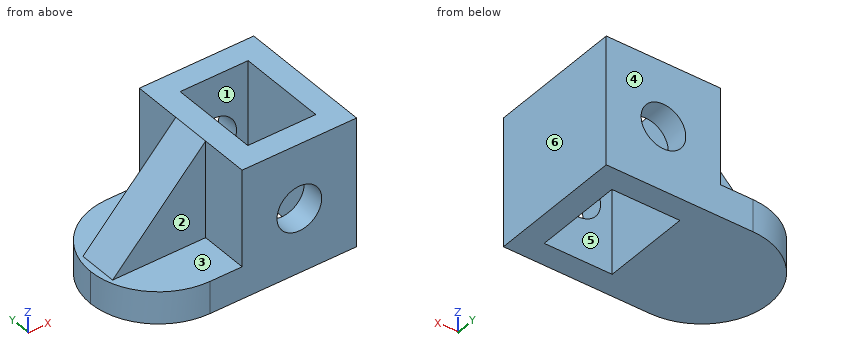
```python
from build123d import *

# Parameters (mm, degrees)
F0_R     = 12.5
F1_DEPTH = 76
F2_W     = 38
F2_H     = 50
F3_DEPTH = 124
F5_DEPTH = 125.4
F7_DEPTH = 54
F9_DEPTH = 25


with BuildPart() as f1:
    # F0 (on Front) → F1 (new body)
    with BuildSketch(Plane.XZ):
        Polygon((0, 18), (0, 0), (120, 0), (120, 72), (56, 72), (56, 18), align=None)
        with Locations((88, 36)):
            Circle(F0_R, mode=Mode.SUBTRACT)
    extrude(amount=F1_DEPTH)

    # F2 (on face) → F3 (cut)
    with BuildSketch(Plane.XY.offset(72)):
        with Locations((88, -38)):
            Rectangle(F2_W, F2_H)
    extrude(amount=-F3_DEPTH, mode=Mode.SUBTRACT)

    # F4 (on face) → F5 (cut)
    with BuildSketch(Plane.XY.offset(18)):
        with BuildLine():
            ThreePointArc((0, -38), (11.129942, -11.129942), (38, 0))
            Line((38, 0), (0, 0))
            Line((0, 0), (0, -38))
        make_face()
        with BuildLine():
            ThreePointArc((38, -76), (11.129942, -64.870058), (0, -38))
            Line((0, -38), (0, -76))
            Line((0, -76), (38, -76))
        make_face()
    extrude(amount=-F5_DEPTH, mode=Mode.SUBTRACT)

    # F6 (on face) → F7 (join)
    with BuildSketch(Plane.XY.offset(18)):
        Polygon((56, -49), (56, -38), (56, -27), (4, -27), (4, -49), align=None)
    extrude(amount=F7_DEPTH)

    # F8 (on face) → F9 (cut)
    with BuildSketch(Plane.XZ.offset(49)):
        Polygon((4, 72), (4, 18), (56, 72), align=None)
    extrude(amount=-F9_DEPTH, mode=Mode.SUBTRACT)


solid = f1.part
```
Input: part model. Units: mm. Frame: model coordinates. Face numbers are marked on the shaded views. A direction names the side the tool comes from. Give positions to 0.01 mm unless a question says otherwise; leave off trailing zeros. Order: outer loops, then holes, each group sorted by start corner. A loop starts at its lowest first (then second) coordinate and runs counter-clockwise, first axis right, second up. Notation, with made-up numbers: M 3,15.5 L 30,15.5 A19 cw 30,33.5 Z; hole C 40,57 d9. An arc over 180 degrees is marked long. One line per question, with ' | ' between items.
1) Draft query along X for the marked faces 4, 5 and 6. Return one class per face: pulls with the +X half, pulls with the -X half, needs draft (parallel to the pull), parting line crosses it, or undercut.
Filled in:
face 4: needs draft | face 5: undercut | face 6: pulls with the +X half
2) Section B-B on z = 16.5. Output: boundary loops of the cut face in (x, y), and give its area (3 significant figures).
Filled in:
outline: M 0,-38 A38 ccw 38,-76 L 120,-76 L 120,0 L 38,0 A38 ccw Z; hole M 69,-63 L 107,-63 L 107,-13 L 69,-13 Z | area: 6,600 mm2
3) Section A-A on x = 88. Output: boundary loops of the cut face in (y, z).
Filled in:
outline: M -76,0 L -63,0 L -63,23.5 L -76,23.5 Z; M -76,48.5 L -63,48.5 L -63,72 L -76,72 Z; M -13,0 L 0,0 L 0,23.5 L -13,23.5 Z; M -13,48.5 L 0,48.5 L 0,72 L -13,72 Z
4) Ray query, L1, parallel to Y at x = 74, z = 48; L2, parallel to Z at x = 88, y = -8.5; L3, parallel to X at y = -70, z = 36. Return the intervals inside material, ascending.
Filled in:
L1: y = -76 to -63, -13 to 0 | L2: z = 0 to 23.5, 48.5 to 72 | L3: x = 56 to 75.5, 100.5 to 120
5) Section D-D on z = 36. Output: boundary loops of the cut face in (x, y), and give its area (3 significant figures).
Filled in:
outline: M 21.33,-49 L 56,-49 L 56,-76 L 75.5,-76 L 75.5,-63 L 69,-63 L 69,-13 L 75.5,-13 L 75.5,0 L 56,0 L 56,-27 L 21.33,-27 Z; M 100.5,-76 L 120,-76 L 120,0 L 100.5,0 L 100.5,-13 L 107,-13 L 107,-63 L 100.5,-63 Z | area: 3,080 mm2
6) Section C-C on y = -58. Output: boundary loops of the cut face in (x, z).
Filled in:
outline: M 5.69,0 L 69,0 L 69,72 L 56,72 L 56,18 L 5.69,18 Z; M 107,0 L 120,0 L 120,72 L 107,72 Z
7) Contact query for flat-ended pins moving along their axis: P1, Ø2, axis at x = 25, y = -39, coming from the +Z side; P2, Ø15, axis at x = 88, z = 36, coming from the +Y side; P3, Ø1.5, axis at y = -48.5, z = 63, coming from the -X side; P4, Ø17, axis at x = 20.5, y = -44, coming from the +Z side. Output: stop coordinate, or through.
Filled in:
P1: stops at z = 40.85 | P2: passes through | P3: stops at x = 46.61 | P4: stops at z = 43.96
8) Access query for the marked faces 1, 2 and 3. Directions: +Z, -Z, +X, -X, +Y, -Y. A direction counts if a zero-diameter tool reaches every point of the face in a straight line with its end or side. Return the directions, or none.
Filled in:
face 1: +Z, -Z | face 2: +Z, -X, -Y | face 3: +Z, -X
